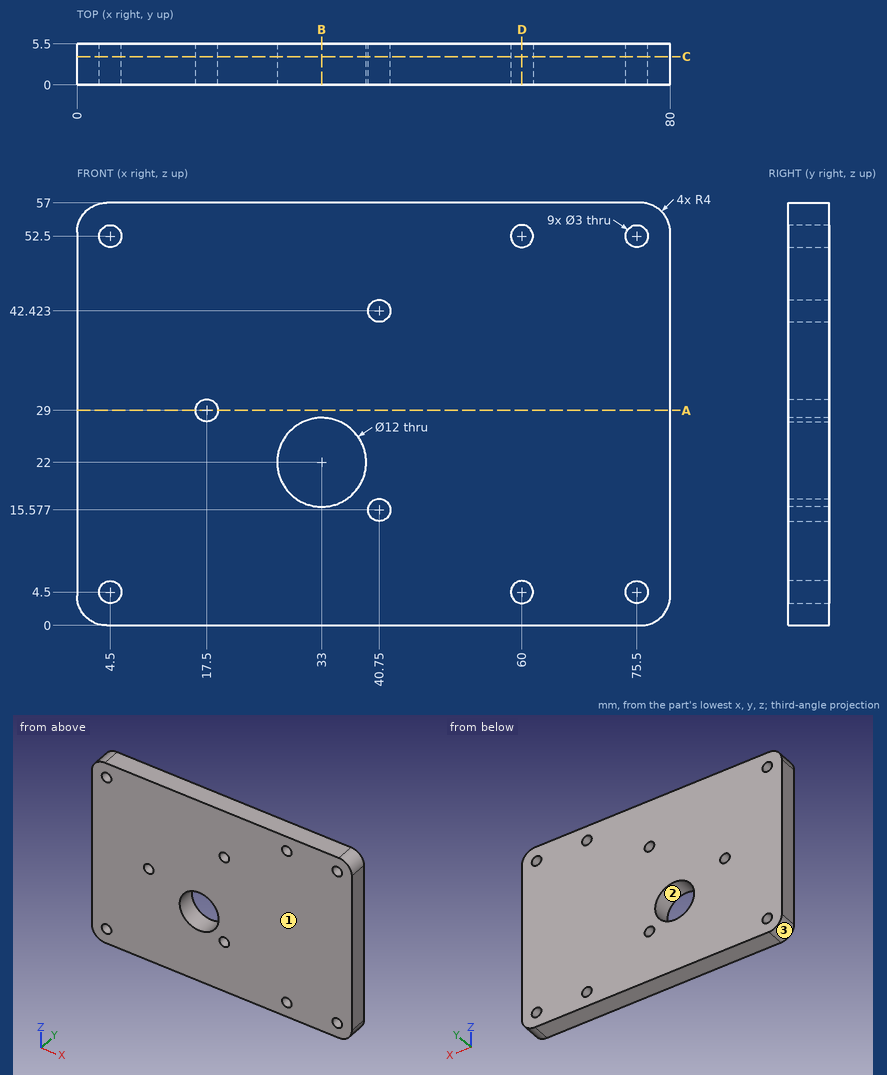
Input: dimensioned drawing with shaded views. Units: mm. Origin: part minimum x, y, z. Round coordinates to 2 decimals unless told otherwise and drop trailing zeros. Loops run counter-clockwise (first coordinate to the right, second up) from the corner with the lowest first, then second, coordinate; pieces in that order, holes last. Notation, with made-up numbers: (22, -29.75) -> (62, -29.75) arc R34 ccw to (62, 4.25) -> close; hole circle Ø8 at (87, 56.5). An arc over 180 degrees is marked (long way). Answer as a JSON object with one key per item and string values. Group by question number.
Q1. Section query B-B (x = 33). Output: boundary loops of the cut face in (y, z).
Q2. Contact query for a flat-ended pin moving along its axis: P1, Ø4, axis at x = 75.5, z = 4.5, coming from the +Y side. Output: stop coordinate, or through.
Q3. Section query C-C (y = 3.8). State how many separate pieces and enclosed holes the cut face has, plus the area to 3 significant figures.
Q4. Section query D-D (x = 60). Output: boundary loops of the cut face in (y, z).
Q5. Mould query, pull axis Z, two halves, no side actions, for the marked faces 1, 2 and 3. Classes: pulls with the +Z half, pulls with the -Z half, needs draft (parallel to the pull), parting line crosses it, or undercut.
Q6. Section query A-A (z = 29). Output: boundary loops of the cut face in (x, y).
Q7. Ray query, line 1 (X direction, y = 1.5, z = 4.5); line 2 (Z direction, x = 75.5, y = 2.5); line 3 (Z direction, x = 17.5, y = 3.25). Return the intervals inside material, ascending. Write a range as from..to.
Completed:
{
 "1": {"outline": "(0, 0) -> (5.5, 0) -> (5.5, 16) -> (0, 16) -> close; (0, 28) -> (5.5, 28) -> (5.5, 57) -> (0, 57) -> close"},
 "2": {"P1": "y = 5.5"},
 "3": {"separate pieces": "1", "enclosed holes": "10", "area": "4,370 mm²"},
 "4": {"outline": "(0, 0) -> (5.5, 0) -> (5.5, 3) -> (0, 3) -> close; (0, 6) -> (5.5, 6) -> (5.5, 51) -> (0, 51) -> close; (0, 54) -> (5.5, 54) -> (5.5, 57) -> (0, 57) -> close"},
 "5": {"face 1": "needs draft", "face 2": "undercut", "face 3": "pulls with the -Z half"},
 "6": {"outline": "(0, 0) -> (16, 0) -> (16, 5.5) -> (0, 5.5) -> close; (19, 0) -> (80, 0) -> (80, 5.5) -> (19, 5.5) -> close"},
 "7": {"line 1": "0..3, 6..58.5, 61.5..74, 77..80", "line 2": "0..3, 6..51, 54..57", "line 3": "0..27.5, 30.5..57"}
}
